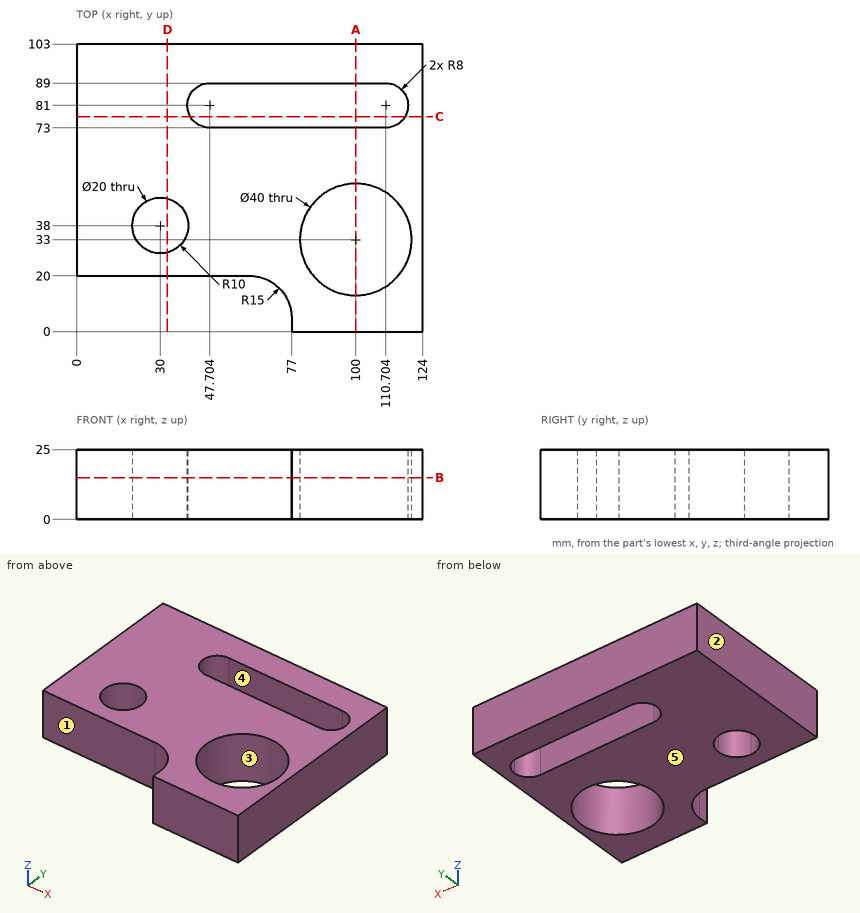
Print and shaded views of the part. All mm, measured from the part's lowest x, y and z. A direction names the side the tool comes from. Give positions to 0.01 mm unless a question says otherwise; leave off trailing zeros. Write each loop counter-clockwise with the first axis right and the second up, starting at its lowest first coordinate (ties: lowest second). Pieces come first, ordered by that corner, then holes. Notation, with made-up numbers: (0.25, 24) - (4.25, 24) arc R22 ccw to (4.25, 59) - close; hole circle Ø5 at (33, 19.25). An arc over 180 degrees is marked (long way). One line per question, with ' | ' between items. Start each with the question number.
(1) Pin check, flat tips, straight feed: P1, Ø5, axis at x = 54, y = 17, coming from the +Z side; P2, Ø1.5, axis at y = 3.5, z = 11.5, coming from the -X side; P3, Ø12.5, axis at x = 69, z = 10, coming from the -Y side; P4, Ø12.5, axis at x = 17, z = 17, coming from the -Y side. Stop position of each tip, or through.
(2) Two-plate mould, pull along X, no slides. Class the marked faces 1, 2 and 3: +X half, -X half, draft (parallel to the pull), parting line (faces both ways), or undercut.
(3) Slice it at B-B on z = 15. Write the cut outline in (x, y), plus the area to 3 significant figures.
(4) 3-axis set-ups, long thin cutter, end or side, ignore diameter. For the marked faces 4 and 5: which of +Z, -Z, +X, -X, +Y, -Y reach the whole face in a straight line?
(5) Slice it at C-C on y = 77. Write the cut outline in (x, z), plus the area to 3 significant figures.
(6) Slice it at A-A on x = 100. Write the cut outline in (y, z).
(7) Wall check: line 1 along Y through (x, z) = (100, 17.25); line 2 along X through (y, z) = (30.5, 16.75) (1 decimal); line 3 along Y through (x, z) = (92, 18.5). Give the ranges that are in metal, low to high. Write a range as from..to.
(8) Slice it at D-D on x = 32.5. Write the cut outline in (y, z), plus the area to 3 significant figures.
Results below:
1) P1: through | P2: x = 77 | P3: y = 12.03 | P4: y = 20
2) face 1: draft | face 2: -X half | face 3: undercut
3) outline: (0, 20) - (62, 20) arc R15 cw to (77, 5) - (77, 0) - (124, 0) - (124, 103) - (0, 103) - close; hole (30, 28) arc R10 ccw to (40, 38) arc R10 ccw (long way) to start; hole (39.7, 81) arc R8 ccw to (47.7, 73) - (110.7, 73) arc R8 ccw to (118.7, 81) arc R8 ccw to (110.7, 89) - (47.7, 89) arc R8 ccw to start; hole circle Ø40 at (100, 33) | area: 8,500 mm^2
4) face 4: +Z, -Z | face 5: -Z, +X, -X, +Y, -Y
5) outline: (0, 0) - (40.78, 0) - (40.78, 25) - (0, 25) - close; (117.63, 0) - (124, 0) - (124, 25) - (117.63, 25) - close | area: 1,180 mm^2
6) outline: (0, 0) - (13, 0) - (13, 25) - (0, 25) - close; (53, 0) - (73, 0) - (73, 25) - (53, 25) - close; (89, 0) - (103, 0) - (103, 25) - (89, 25) - close
7) line 1: 0..13, 53..73, 89..103 | line 2: 0..23.4, 36.6..80.2, 119.8..124 | line 3: 0..14.67, 51.33..73, 89..103
8) outline: (20, 0) - (28.32, 0) - (28.32, 25) - (20, 25) - close; (47.68, 0) - (103, 0) - (103, 25) - (47.68, 25) - close | area: 1,590 mm^2
